```python
from build123d import *

# Parameters (mm, degrees)
F1_DEPTH = 25
F4_DEPTH = 5
F5_R     = 12.49999
F6_R     = 2


# Not quite as in the source:
# - a fillet or chamfer is up to 0.001 mm smaller than in the source, because OpenCascade refuses the exact size


with BuildPart() as f1:
    # F0 (on Right) → F1 (new body)
    with BuildSketch(Plane.YZ):
        Polygon((0, 300), (0, 0), (350, 0), (350, 5), (5, 5), (5, 300), align=None)
    extrude(amount=-F1_DEPTH)

    # F3 (on offset) → F4 (join)
    with BuildSketch(Plane.YZ.offset(-10)):
        Polygon((10, 250), (5, 250), (5, 5), (300, 5), (300, 10), (20, 20), align=None)
    extrude(amount=-F4_DEPTH)

    # F5 (radius 12.5 in the source; OpenCascade refuses exactly that, so slightly less here)
    f5_edges = [f1.edges().sort_by_distance(p)[0] for p in [
        (0, 2.5, 300),
        (-25, 2.5, 300),
        (-25, 350, 2.5),
        (0, 350, 2.5),
        (-12.5, 20, 20),
    ]]
    fillet(f5_edges, radius=F5_R)

    # F6
    f6_edges = [f1.edges().sort_by_distance(p)[0] for p in [
        (0, 5, 146.250005),
        (-3.661162, 5, 296.338838),
        (-5, 5, 5),
        (-12.5, 5, 300),
        (-10, 5, 127.5),
        (-21.338838, 5, 296.338838),
        (-12.5, 5, 250),
        (-25, 5, 146.250005),
        (-15, 5, 127.5),
        (-20, 5, 5),
        (-10, 14.749198, 140.768451),
        (-12.5, 19.498396, 31.536902),
        (-12.5, 10, 250),
        (-15, 14.749198, 140.768451),
        (-15, 165.770222, 14.793921),
        (-15, 23.182084, 23.206847),
        (-15, 300, 7.5),
        (-15, 152.5, 5),
        (-15, 7.5, 250),
        (-10, 165.770222, 14.793921),
        (-10, 23.182084, 23.206847),
        (-10, 300, 7.5),
        (-10, 152.5, 5),
        (-10, 7.5, 250),
        (0, 171.250005, 5),
        (-3.661162, 346.338838, 5),
        (-12.5, 350, 5),
        (-21.338838, 346.338838, 5),
        (-12.5, 300, 5),
        (-25, 171.250005, 5),
        (-12.5, 300, 10),
    ]]
    fillet(f6_edges, radius=F6_R)


solid = f1.part
```
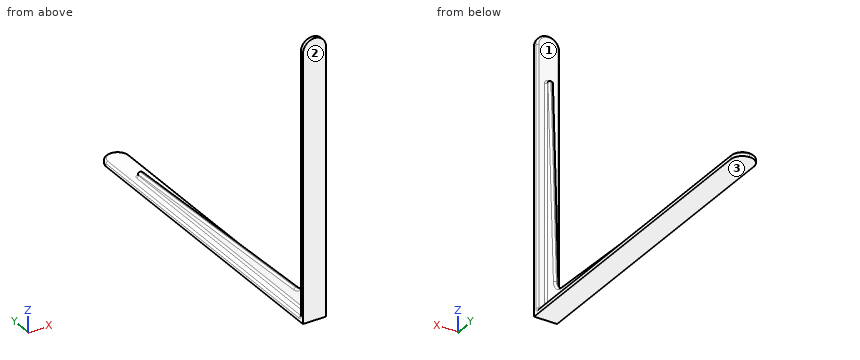
Input: part model. Units: mm. Frame: model coordinates. Face numbers are marked on the shaded views. Give positions to 0.01 mm unless a question says otherwise; leave off trailing zeros. Order: outer loops, then holes, each group sorted by start corner. A loop starts at its lowest first (then second) coordinate and runs counter-clockwise, first axis right, second up. Notation, with made-up numbers: (-31.75, 26) - (4.25, 26) arc R24 cw to (4.25, 45) - close; hole circle Ø1 at (89.25, 85.25). An arc over 180 degrees is marked (long way). Use a Markdown table: item, result.
(1) Draft query along Y for the marked faces 1, 2 and 3. Return one class per face: released by +Y, released by -Y, zero draft, split by the parting line, or undercut.
Computed values:
| item | result |
|---|---|
| face 1 | released by +Y |
| face 2 | released by -Y |
| face 3 | zero draft |
(2) Line query: line 1 (Z direction, x = -19.75, y = 101); line 2 (Z direction, x = -9.25, y = 66). Output: solid intervals per line, ascending. Write a range as from..to.
Computed values:
| item | result |
|---|---|
| line 1 | z = 0..5 |
| line 2 | z = 0..5.44 |
(3) Pin query (flat end, axial travel): pin 1 (1 mm diameter, centred on x = -6.5, z = 185.5, fed in from +Y); pin 2 (0.8 mm diameter, centred on x = -12.5, y = 7.5, fed in from +Z); pin 3 (5 mm diameter, centred on x = -3.5, z = 187.5, fed in from -Y); pin 4 (0.8 mm diameter, centred on x = -12.5, z = 7.5, fed in from +Y). Return the tip coordinate at first contact, or that it passes through.
Computed values:
| item | result |
|---|---|
| pin 1 | stops at y = 5 |
| pin 2 | stops at z = 250 |
| pin 3 | stops at y = 0 |
| pin 4 | stops at y = 300 |
(4) Section query A-A (z = 262). Output: boundary loops of the cut face in (x, y), then the cut area to 3 significant figures.
Computed values:
| item | result |
|---|---|
| outline | (-25, 0) - (0, 0) - (0, 3) arc R2 ccw to (-2, 5) - (-23, 5) arc R2 ccw to (-25, 3) - close |
| area | 123 mm2 |
